For this review, take the finished solid that the model builds, in its own axes (mm). Face numbers are marked on the shaded views. A direction names the side the tool comes from. Round coordinates to 2 decimals unless told otherwise and drop trailing zeros. Order: outer loops, then holes, each group sorted by start corner. A loop starts at its lowest first (then second) coordinate and runs counter-clockwise, first axis right, second up. Notation, with made-up numbers: (-18, 89) - (28, 89) arc R32 ccw to (28, 115) - close; hole circle Ø11 at (39.5, -26.5). An arc over 180 degrees is marked (long way). One line per question, with ' | ' between items.
Autodesk Inventor part; units mm, degrees
ref_plane "YZ Plane" through (0, 0, 0) normal (1, 0, 0) x (0, 1, 0)
ref_plane "XZ Plane" through (0, 0, 0) normal (0, 1, 0) x (-1, 0, 0)
ref_plane "XY Plane" through (0, 0, 0) normal (0, 0, 1) x (1, 0, 0)
sketch "Sketch1" plane through (0, 0, 0) normal (0, 1, 0) x (-1, 0, 0)
  line L0 (0, 11.547) -> (10, 5.7735)
  line L1 (10, 5.7735) -> (10, -5.7735)
  line L2 (10, -5.7735) -> (0, -11.547)
  line L3 (0, -11.547) -> (-10, -5.7735)
  line L4 (-10, -5.7735) -> (-10, 5.7735)
  line L5 (-10, 5.7735) -> (0, 11.547)
  line L6 (-10, 5.7735) -> (-20, 11.547)
  line L7 (-20, 11.547) -> (-20, 23.094)
  line L8 (-20, 23.094) -> (-10, 28.8675)
  line L9 (-10, 28.8675) -> (0, 23.094)
  line L10 (0, 23.094) -> (0, 11.547)
  line L11 (0, 11.547) -> (-10, 5.7735)
  circle A0 centre (-15.1962, 2.7735) radius 1.6
  circle A1 centre (5.1962, 14.547) radius 1.6
  line L12 (0, 11.547) -> (5.1962, 14.547)
  line L13 (-10, 5.7735) -> (-15.1962, 2.7735)
  line L14 (-10, 5.7735) -> (-10, -0.2265)
  line L15 (-10, -0.2265) -> (-15.1962, -3.2265)
  line L16 (-15.1962, -3.2265) -> (-20.3923, -0.2265)
  line L17 (-20.3923, -0.2265) -> (-20.3923, 5.7735)
  line L18 (-20.3923, 5.7735) -> (-15.1962, 8.7735)
  line L19 (-15.1962, 8.7735) -> (-10, 5.7735)
  line L20 (0, 11.547) -> (0, 17.547)
  line L21 (0, 17.547) -> (5.1962, 20.547)
  line L22 (5.1962, 20.547) -> (10.3923, 17.547)
  line L23 (10.3923, 17.547) -> (10.3923, 11.547)
  line L24 (10.3923, 11.547) -> (5.1962, 8.547)
  line L25 (5.1962, 8.547) -> (0, 11.547)
  dimension "d26" = 3.2
  dimension "d27" = 3.2
  dimension "d28" = 6
  dimension "d29" = 6
extrude "Extrusion1" add sketch "Sketch1" along normal blind 3
properties part number "Dribbler Plate" material "Polycarbonate, Smoke"
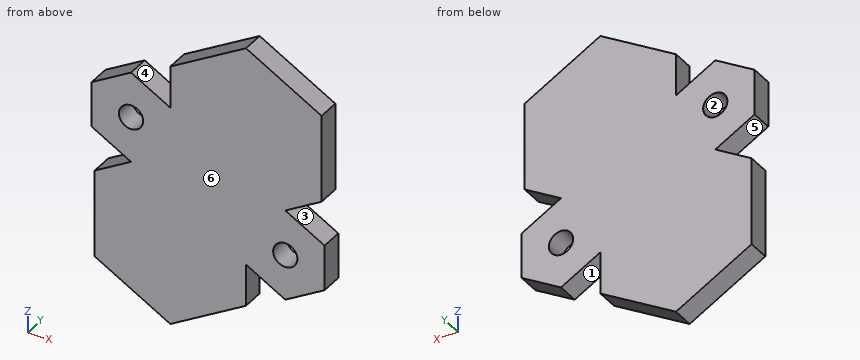
(1) We need section D-D on x = -3. State the section outline as (y, z) points, plus the area to 3 significant figures.
Output values:
outline: (0, -9.81) - (3, -9.81) - (3, 19.28) - (0, 19.28) - close | area: 87.3 mm^2
(2) Insertion check: pin 1 (0.9 mm diameter, centred on y = 2, z = 19.5, fed in from -X); pin 2 (1 mm diameter, centred on y = 1.5, z = 12, fed in from +X); pin 3 (3 mm diameter, centred on x = 15.2, z = 2.77, fed in from +Y); pin 4 (1.5 mm diameter, centred on x = 4, y = 2, fed in from +Z). Each pin has a flat end and moves straight along its axis. Give the tip position at first contact, or say it passes through.
Output values:
pin 1: x = -7.79 | pin 2: x = 20 | pin 3: through | pin 4: z = 25.84
(3) Mouldability with a two-part tool opening along Z and no side actions: class the marked faces 4, 5 and 6 as released by +Z, released by -Z, zero draft, split by the parting line, or undercut.
Output values:
face 4: released by +Z | face 5: undercut | face 6: zero draft
(4) For probe 1 along Z at (x, y) = (-6, 2.1); probe 2 along X at (y, z) = (0.95, 21); probe 3 along X at (y, z) = (2.1, 12), list the stretches that pass through material, from the lowest coordinate up. Write a range as [from, to].
Output values:
probe 1: [-8.08, 8.08], [9.01, 13.16], [15.93, 20.08] | probe 2: [0, 20] | probe 3: [-10.39, 20]
(5) We need section A-A on z = 15. State the section outline as (x, y) points, plus the area to 3 significant figures.
Output values:
outline: (-10.39, 0) - (-6.73, 0) - (-6.73, 3) - (-10.39, 3) - close; (-3.66, 0) - (20, 0) - (20, 3) - (-3.66, 3) - close | area: 82.0 mm^2
(6) We need section B-B on y = 0.85. State the section outline as (x, z) points.
Output values:
outline: (-10.39, 11.55) - (-5.2, 8.55) - (-10, 5.77) - (-10, -5.77) - (0, -11.55) - (10, -5.77) - (10, -0.23) - (15.2, -3.23) - (20.39, -0.23) - (20.39, 5.77) - (15.2, 8.77) - (20, 11.55) - (20, 23.09) - (10, 28.87) - (0, 23.09) - (0, 17.55) - (-5.2, 20.55) - (-10.39, 17.55) - close; hole circle Ø3.2 at (-5.2, 14.55); hole circle Ø3.2 at (15.2, 2.77)
(7) For the marked faces 1, 2 and 3, list the 3-axis set-ups (+Z, -Z, +X, -X, +Y, -Y) from which the entire face can be reached by the end or side of a thin tool; tool diameter is ignored.
Output values:
face 1: -Z, +Y, -Y | face 2: +Y, -Y | face 3: +X, +Y, -Y
(8) We need section C-C on z = 19.5. State the section outline as (x, y) points, plus the area to 3 significant figures.
Output values:
outline: (-7.01, 0) - (-3.38, 0) - (-3.38, 3) - (-7.01, 3) - close; (0, 0) - (20, 0) - (20, 3) - (0, 3) - close | area: 70.9 mm^2
